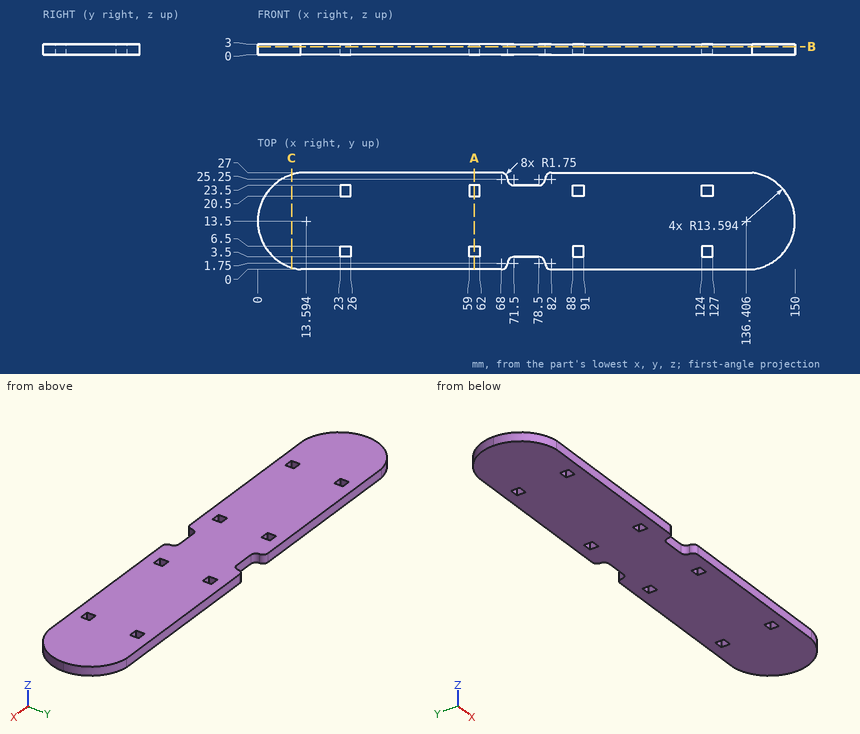
Design review of the part shown in the three views and the two pictorial views. Dimensions are in mm from the part's minimum x, y and z. Round coordinates to 2 decimals unless told otherwise and drop trailing zeros. Loops run counter-clockwise (first coordinate to the right, second up) from the corner with the lowest first, then second, coordinate; pieces in that order, holes last.
1) Wall thickness on line 1 along Y through (x, z) = (60, 1.3); line 2 along X through (y, z) = (4.25, 2.45); line 3 along X through (y, z) = (3.75, 2.55): over which ranges is each line inside the solid? List them lowest first.
Values follow:
line 1: y = 0 to 3.5, 6.5 to 20.5, 23.5 to 27
line 2: x = 3.63 to 23, 26 to 59, 62 to 88, 91 to 124, 127 to 146.37
line 3: x = 4.12 to 23, 26 to 59, 62 to 88, 91 to 124, 127 to 145.88
2) Consider section A-A on x = 60.5. State the section outline as (y, z) points.
Values follow:
outline: (0, 0) - (3.5, 0) - (3.5, 3) - (0, 3) - close; (6.5, 0) - (20.5, 0) - (20.5, 3) - (6.5, 3) - close; (23.5, 0) - (27, 0) - (27, 3) - (23.5, 3) - close
3) Consider section C-C on x = 9.5. State the section outline as (y, z) points.
Values follow:
outline: (0.54, 0) - (26.46, 0) - (26.46, 3) - (0.54, 3) - close
4) Clearance check with flat-ended pins moving along their axes: P1, Ø1, axis at x = 71.5, z = 2.5, coming from the +Y side; P2, Ø1.5, axis at y = 21.5, z = 2, coming from the -X side (1 decimal); P3, Ø1.5, axis at x = 74.5, z = 1, coming from the +Y side. State where each tip first meets the part, or that it passes through.
Values follow:
P1: stops at y = 23.57
P2: stops at x = 2.1
P3: stops at y = 23.5
5) Consider section B-B on z = 2.3. Give the number of separate pieces and of enclosed holes in the cut face, then the cut area to 3 significant figures.
Values follow:
separate pieces: 1
enclosed holes: 8
area: 3,750 mm2
